The model under review builds one solid part; all positions refer to its coordinate system, in mm. Give positions to 0.01 mm unless a question says otherwise; leave off trailing zeros. Write each loop counter-clockwise with the first axis right and the second up, starting at its lowest first coordinate (ties: lowest second). Pieces come first, ordered by that corner, then holes.
from build123d import *

# Parameters (mm, degrees)
SKETCH1_R           = 20
SKETCH1_R_2         = 15
BOSS_EXTRUDE1_DEPTH = 22


with BuildPart() as part:
    # Sketch1 → Boss-Extrude1 (new, symmetric)
    with BuildSketch(Plane.XY):
        with BuildLine():
            ThreePointArc((29.974824802, 99.228770963), (0, 128), (-29.974824802, 99.228770963))
            ThreePointArc((-29.974824802, 99.228770963), (-44.809013245, 56.006438032), (-80.883915711, 27.95604369))
            ThreePointArc((-80.883915711, 27.95604369), (-99.085824928, 7.349475372), (-92.857575187, -19.430163575))
            ThreePointArc((-92.857575187, -19.430163575), (-76.859583983, -49.370140698), (-74.716930719, -83.248555502))
            ThreePointArc((-74.716930719, -83.248555502), (-64.373950523, -107.45457275), (-38.095238095, -108.983553944))
            ThreePointArc((-38.095238095, -108.983553944), (0, -99.330926563), (38.095238095, -108.983553944))
            ThreePointArc((38.095238095, -108.983553944), (64.373950523, -107.45457275), (74.716930719, -83.248555502))
            ThreePointArc((74.716930719, -83.248555502), (76.859583983, -49.370140698), (92.857575187, -19.430163575))
            ThreePointArc((92.857575187, -19.430163575), (99.085824928, 7.349475372), (80.883915711, 27.95604369))
            ThreePointArc((80.883915711, 27.95604369), (44.809013245, 56.006438032), (29.974824802, 99.228770963))
        make_face()
        with Locations((0, 98)):
            Circle(SKETCH1_R, mode=Mode.SUBTRACT)
        with Locations((70, 0)):
            Circle(SKETCH1_R, mode=Mode.SUBTRACT)
        with Locations((-70, 0)):
            Circle(SKETCH1_R, mode=Mode.SUBTRACT)
        with Locations((50, -87)):
            Circle(SKETCH1_R_2, mode=Mode.SUBTRACT)
        with Locations((-50, -87)):
            Circle(SKETCH1_R_2, mode=Mode.SUBTRACT)
    extrude(amount=BOSS_EXTRUDE1_DEPTH, both=True)


solid = part.part
1) To check wall thickness, follow probe 1 along Y at (x, z) = (-58.5, 2.5); probe 2 along X at (y, z) = (-84, -15); probe 3 along Y at (x, z) = (17, -10). State the ranges of each line that lie inside material, in increasing order.
2) Insertion check: pin 1 (3 mm diameter, centred on x = -24, z = -2.5, fed in from -Y); pin 2 (10 mm diameter, centred on x = -23, z = -0.5, fed in from +Y); pin 3 (10 mm diameter, centred on x = 1.5, z = 4.5, fed in from -Y). Each pin has a flat end and moves straight along its axis. Give the tip position at first contact, or say it passes through.
3) Consider section A-A, the plane y = 0. Give the boundary of the cut face in (x, z), then the cut area to 3 significant figures.
4) Consider section B-B, the plane x = 0. Give the boundary of the cut face in (y, z).
5) Consider section D-D, the plane z = 1.5. Give the boundary of the cut face in (x, y), then the cut area to 3 significant figures.
6) Consider section C-C, the plane x = -61. Give the boundary of the cut face in (y, z), then the cut area to 3 significant figures.
7) The part is to be moulded in two halves that separate along Y. For faces 1 (the cylindrical face through (76.73, -49.83, 0.31)), 2 (the cylindrical face through (50.02, 0.88, -0.31)), 3 (the cylindrical face through (0.642, 127.993, 0.308)), 4 (the flat face through (-1, -17, 22)), say which applies: +Y half, -Y half, draft (parallel to the pull), parting line (faces both ways), or undercut.
Answer block:
1. probe 1: y = -110.51 to -99.36, -74.64 to -16.36, 16.36 to 41.21
1. probe 2: x = -74.82 to -64.7, -35.3 to 35.3, 64.7 to 74.82
1. probe 3: y = -101.16 to 87.46, 108.54 to 122.72
2. pin 1: stops at y = -103.5
2. pin 2: stops at y = 122
2. pin 3: stops at y = -99.6
3. outline: (-100, -22) - (-90, -22) - (-90, 22) - (-100, 22) - close; (-50, -22) - (50, -22) - (50, 22) - (-50, 22) - close; (90, -22) - (100, -22) - (100, 22) - (90, 22) - close
3. area: 5,280 mm2
4. outline: (-99.33, -22) - (78, -22) - (78, 22) - (-99.33, 22) - close; (118, -22) - (128, -22) - (128, 22) - (118, 22) - close
5. outline: (-92.86, -19.43) arc R80 cw to (-74.72, -83.25) arc R25 ccw to (-38.1, -108.98) arc R80 cw to (38.1, -108.98) arc R25 ccw to (74.72, -83.25) arc R80 cw to (92.86, -19.43) arc R30 ccw to (80.88, 27.96) arc R80 cw to (29.97, 99.23) arc R30 ccw to (-29.97, 99.23) arc R80 cw to (-80.88, 27.96) arc R30 ccw to start; hole circle Ø40 at (-70, 0); hole circle Ø30 at (-50, -87); hole circle Ø40 at (0, 98); hole circle Ø30 at (50, -87); hole circle Ø40 at (70, 0)
5. area: 24,900 mm2
6. outline: (-109.45, -22) - (-97.2, -22) - (-97.2, 22) - (-109.45, 22) - close; (-76.8, -22) - (-17.86, -22) - (-17.86, 22) - (-76.8, 22) - close; (17.86, -22) - (39.2, -22) - (39.2, 22) - (17.86, 22) - close
6. area: 4,070 mm2
7. face 1: undercut
7. face 2: undercut
7. face 3: +Y half
7. face 4: draft
